Can you work these out from the drawing? Everything is in mm from the part's minimum corner. Round coordinates to 2 decimals unless told otherwise and drop trailing zeros. Loops run counter-clockwise (first coordinate to the right, second up) from the corner with the lowest first, then second, coordinate; pieces in that order, holes last. Notation, with made-up numbers: (50, -24.5) -> (71, -24.5) arc R30 ccw to (71, 9.5) -> close; hole circle Ø7 at (-32, 17). An arc over 180 degrees is marked (long way). One line per item, written item: value.
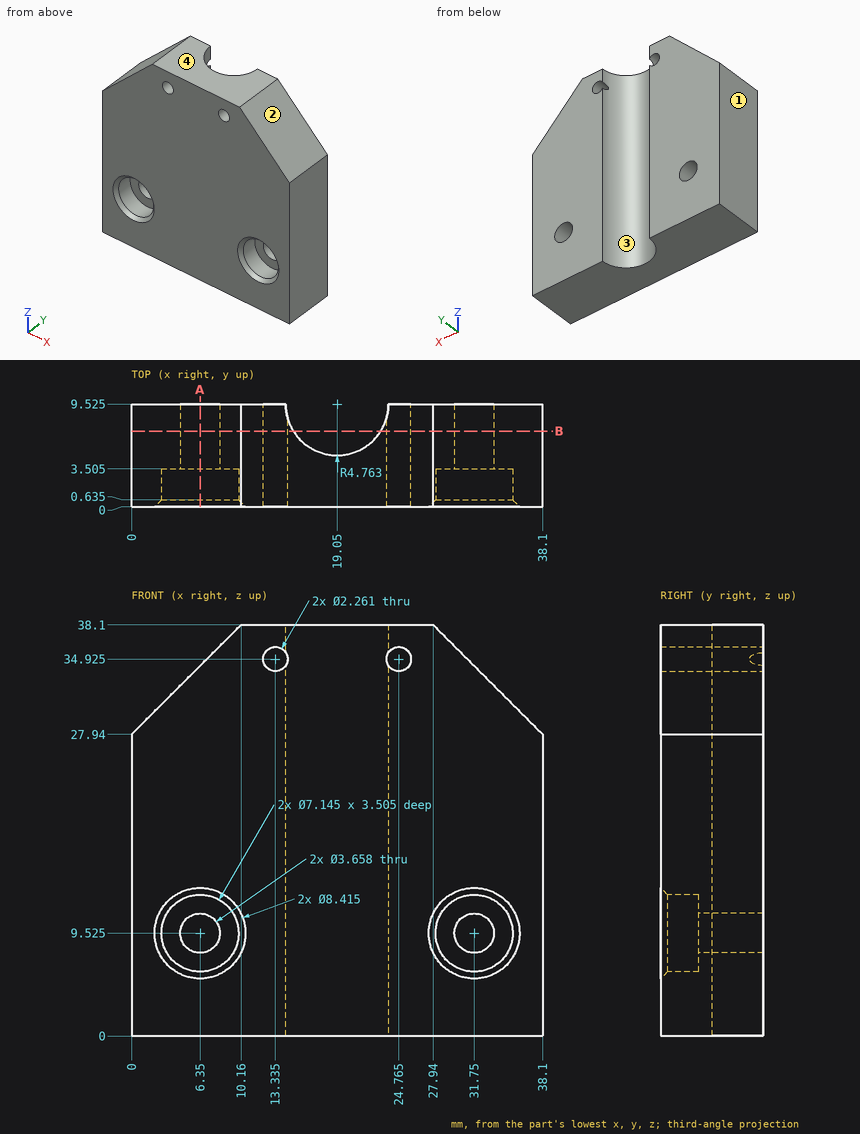
(1) If I drill on L1, parallel to X at y = 8.25, z = 12.5; L2, parallel to X at y = 1.5, z = 6.5; L3, parallel to X at y = 2, z = 8, over which ranges is the centre line in solid material (lowest first)?
Recorded:
L1: 0 to 14.46, 23.64 to 38.1
L2: 0 to 4.45, 8.25 to 29.85, 33.65 to 38.1
L3: 0 to 3.12, 9.58 to 28.52, 34.98 to 38.1
(2) I'm going to push flat-ended pins straight in: pin 1 Ø5.5 at (x, z) = (32, 9.5) entering from -Y (1 decimal); pin 2 Ø1 at (x, y) = (7, 6) entering from +Z. Where does each tip first touch, or does it pass through?
Recorded:
pin 1: y = 3.5
pin 2: z = 35.44
(3) If we section it at A-A, the plane x = 6.35: Please give me the cut outline in (y, z) (1 decimal).
Recorded:
outline: (0, 0) -> (9.5, 0) -> (9.5, 7.7) -> (3.5, 7.7) -> (3.5, 6) -> (0.6, 6) -> (0, 5.3) -> close; (0, 13.7) -> (0.6, 13.1) -> (3.5, 13.1) -> (3.5, 11.4) -> (9.5, 11.4) -> (9.5, 34.3) -> (0, 34.3) -> close
(4) If we section it at B-B, the plane y = 7: Give the number of separate pieces and of enclosed holes in the cut face, then the cut area to 3 significant figures.
Recorded:
separate pieces: 2
enclosed holes: 4
area: 1,010 mm²
(5) Thinking about a two-plate mould opening in X: for the marked faces 1, 2, 3 and 4, which applies, released by +X, released by -X, zero draft, split by the parting line, or undercut?
Recorded:
face 1: released by -X
face 2: released by +X
face 3: undercut
face 4: zero draft
